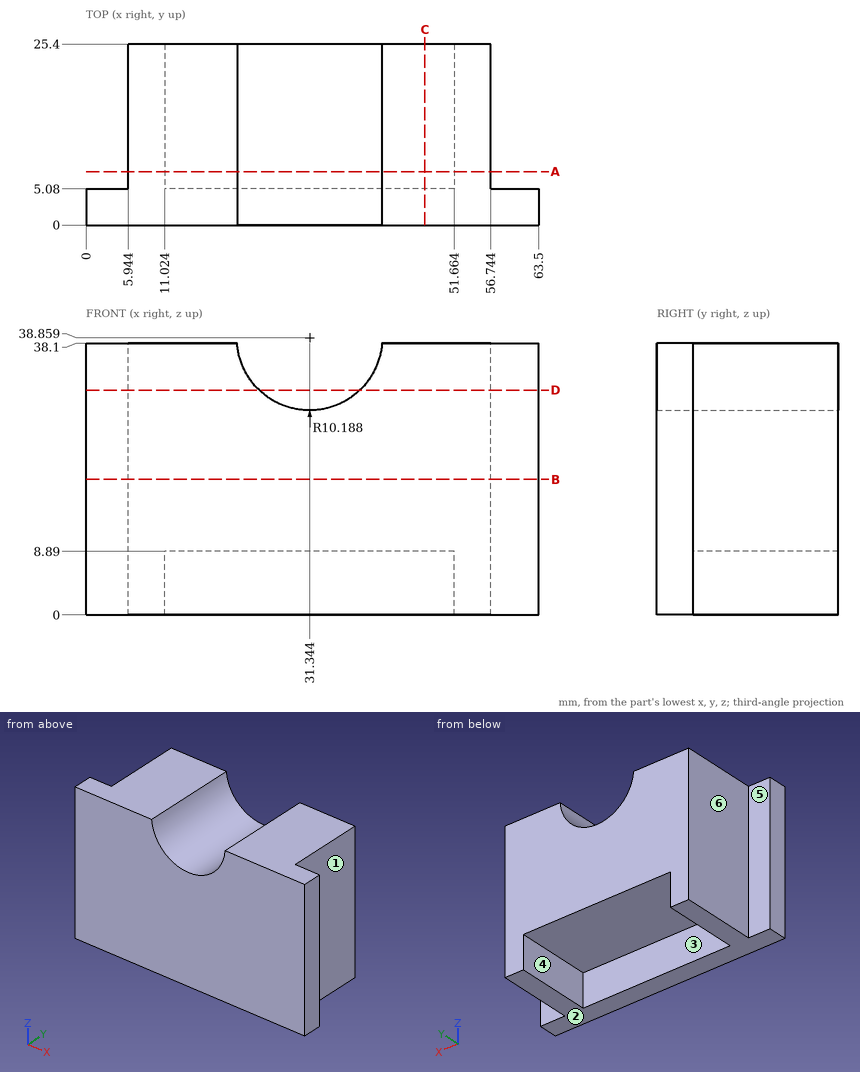
Design review of the part shown in the three views and the two pictorial views. Dimensions are in mm from the part's minimum x, y and z. A direction names the side the tool comes from. Round coordinates to 2 decimals unless told otherwise and drop trailing zeros. Loops run counter-clockwise (first coordinate to the right, second up) from the corner with the lowest first, then second, coordinate; pieces in that order, holes last. Notation, with made-up numbers: (6, 6) -> (55, 6) arc R17 cw to (55, 36) -> close; hole circle Ø2 at (88.25, 85.5). An arc over 180 degrees is marked (long way). Use one line per item in the form item = value. Start each with the question number.
Q1. For pin 1 Ø10 at (x, y) = (41.5, 7.5) entering from -Z; pin 2 Ø6 at (y, z) = (11, 25) entering from -X; pin 3 Ø10 at (y, z) = (15.5, 6.5) entering from +X; pin 4 Ø5.5 at (x, z) = (60, 25.5) entering from +Y, all flat-tipped, find the tip position at first contact; note any pin that passes through.
Q2. We need section D-D on z = 31.5. Give the boundary of the cut face in (x, y) (1 decimal).
Q3. Machinability: for the marked faces 1, 2 and 3, which of the approach directions +Z, -Z, +X, -X, +Y, -Y give a long, thin tool a straight path to every point of the face, cutting with its end or side? Answer none if there is none.
Q4. We need section A-A on y = 7.5. Give the boundary of the cut face in (x, z) (1 decimal), then the cut area to 3 significant figures.
Q5. We need section C-C on x = 47.5. Give the boundary of the cut face in (y, z), then the cut area to 3 significant figures.
Q6. We need section B-B on z = 19. Give the boundary of the cut face in (x, y) (1 decimal), then the cut area to 3 significant figures.
Q7. Wall thickness on line 1 along X through (y, z) = (12.25, 3.5) (1 decimal); line 2 along Z through (x, y) = (21, 18.5); line 3 along X through (y, z) = (23.75, 13) (1 decimal): over which ranges is each line inside the solid? List them lowest first. Write a range as [from, to].
Q8. Draft analysis for pull direction X (two halves, no side actions). For the marked faces 4, 5 and 6, state which applies: +X half, -X half, draft (parallel to the pull), parting line (faces both ways), or undercut.
Calculated:
q1.pin_1 = 0
q1.pin_2 = 5.94
q1.pin_3 = 56.74
q1.pin_4 = 5.08
q2.outline = (0, 0) -> (24.3, 0) -> (24.3, 25.4) -> (5.9, 25.4) -> (5.9, 5.1) -> (0, 5.1) -> close; (38.4, 0) -> (63.5, 0) -> (63.5, 5.1) -> (56.7, 5.1) -> (56.7, 25.4) -> (38.4, 25.4) -> close
q3.face_1 = +Z, -Z, +X, +Y
q3.face_2 = -Z, +X, -X, +Y, -Y
q3.face_3 = -Z, +Y
q4.outline = (5.9, 0) -> (11, 0) -> (11, 8.9) -> (51.7, 8.9) -> (51.7, 0) -> (56.7, 0) -> (56.7, 38.1) -> (41.5, 38.1) arc R10.2 cw to (21.2, 38.1) -> (5.9, 38.1) -> close
q4.area = 1,430 mm²
q5.outline = (0, 0) -> (5.08, 0) -> (5.08, 8.89) -> (25.4, 8.89) -> (25.4, 38.1) -> (0, 38.1) -> close
q5.area = 787 mm²
q6.outline = (0, 0) -> (63.5, 0) -> (63.5, 5.1) -> (56.7, 5.1) -> (56.7, 25.4) -> (5.9, 25.4) -> (5.9, 5.1) -> (0, 5.1) -> close
q6.area = 1,350 mm²
q7.line_1 = [5.9, 11], [51.7, 56.7]
q7.line_2 = [8.89, 38.1]
q7.line_3 = [5.9, 56.7]
q8.face_4 = undercut
q8.face_5 = draft
q8.face_6 = -X half
